from build123d import *

# Parameters (mm, degrees)
F0_R      = 25.4
F1_DEPTH  = 38.1
F3_R      = 4.1275
F4_DEPTH  = 20.0914
F5_R      = 3.4925
F6_DEPTH  = 18.0096
F7_W      = 5.08
F7_H      = 26.67
F8_DEPTH  = 5.08
F9_R      = 25.4
F9_R_2    = 4.1275
F10_DEPTH = 6.35
F11_R     = 25.4
F11_R_2   = 5.3975
F12_DEPTH = 12.7
F13_R     = 2.54
F14_DEPTH = 25.4
F16_R     = 22.225
F16_R_2   = 6.35
F17_DEPTH = 44.45


with BuildPart() as f1:
    # F0 (on Top) → F1 (new body)
    with BuildSketch(Plane.XY):
        Circle(F0_R)
    extrude(amount=-F1_DEPTH)

    # F3 (on face) → F4 (cut)
    with BuildSketch(Plane.XY):
        Circle(F3_R)
    extrude(amount=-F4_DEPTH, mode=Mode.SUBTRACT)

    # F5 (on face) → F6 (cut, through all)
    with BuildSketch(Plane.XY.offset(-20.0914)):
        Circle(F5_R)
    extrude(amount=-F6_DEPTH, mode=Mode.SUBTRACT)

    # F7 (on face) → F8 (cut)
    with BuildSketch(Plane(origin=(0, 0, -38.1), x_dir=(1, 0, 0), z_dir=(0, 0, -1))):
        with Locations((0, -13.335)):
            Rectangle(F7_W, F7_H)
    extrude(amount=-F8_DEPTH, mode=Mode.SUBTRACT)

    # F9 (on face) → F10 (join)
    with BuildSketch(Plane.XY):
        Circle(F9_R)
        Circle(F9_R_2, mode=Mode.SUBTRACT)
    extrude(amount=F10_DEPTH)

    # F11 (on face) → F12 (join)
    with BuildSketch(Plane.XY.offset(6.35)):
        Circle(F11_R)
        Circle(F11_R_2, mode=Mode.SUBTRACT)
    extrude(amount=F12_DEPTH)

    # F13 (on offset) → F14 (cut, through all)
    with BuildSketch(Plane.XZ.offset(-25.4)):
        with Locations((0, 1.524)):
            Circle(F13_R)
    extrude(amount=F14_DEPTH, mode=Mode.SUBTRACT)

    # F16 (on offset) → F17 (cut)
    with BuildSketch(Plane(origin=(0, 0, -31.75), x_dir=(1, 0, 0), z_dir=(0, 0, -1))):
        Circle(F16_R)
        Circle(F16_R_2, mode=Mode.SUBTRACT)
    extrude(amount=-F17_DEPTH, mode=Mode.SUBTRACT)


solid = f1.part
Read the model definition and answer for the solid it produces. Units are mm, in the model's axes. A direction names the side the tool comes from. Give positions to 0.01 mm unless a question says otherwise; leave off trailing zeros. Loops run counter-clockwise (first coordinate to the right, second up) from the corner with the lowest first, then second, coordinate; pieces in that order, holes last. Notation, with made-up numbers: (-36.75, 28.5) -> (21.25, 28.5) arc R8 ccw to (21.25, 38.5) -> close; hole circle Ø1 at (-18.75, 26). An arc over 180 degrees is marked (long way). Use a Markdown table: item, result.
Q1. A tool of negligible diameter and unlimited length cuts with its end or side. For faces 1 (the face through (2.346, 4.825, 0.551)), 2 (the face through (21.199, -6.676, -9.836)), 3 (the face through (2, -4, 6.35)), 4 (the face through (-0.8, -3.4, -29)), 5 (the face through (-2.54, 14, -36)), from which of +Z, -Z, +X, -X, +Y, -Y can it reach the whole face along a straight path? Write none if from no direction.
Solved:
| item | result |
|---|---|
| face 1 | +Y |
| face 2 | none |
| face 3 | +Z |
| face 4 | +Z, -Z |
| face 5 | -Z, +Y |
Q2. Determine the mould class of faces 6 (the face through (0, -5, -38.1)), 7 (the face through (0, 14, -33.02)), 8 (the face through (-5.506, -24.796, -9.925)) for opening direction X: pulls with the +X half, pulls with the -X half, needs draft (parallel to the pull), parting line crosses it, or undercut.
Solved:
| item | result |
|---|---|
| face 6 | needs draft |
| face 7 | undercut |
| face 8 | parting line crosses it |
Q3. Section D-D, the plane y = -10.5 is taken. Determine the outline of the cut face in (x, z).
Solved:
| item | result |
|---|---|
| outline | (-23.13, -38.1) -> (23.13, -38.1) -> (23.13, 19.05) -> (-23.13, 19.05) -> close; hole (-19.59, -31.75) -> (19.59, -31.75) -> (19.59, 12.7) -> (-19.59, 12.7) -> close |
Q4. Section A-A, the plane x = 0 is taken. Count the separate pieces of the cut face and the enclosed holes in it, then the cut area to 3 significant figures.
Solved:
| item | result |
|---|---|
| separate pieces | 3 |
| enclosed holes | 1 |
| area | 872 mm^2 |
Q5. Find the intervals of material crossed by line 1 along Z through (x, y) = (-20.5, -4); line 2 along Y through (x, z) = (1.5, -21); line 3 along Z through (x, y) = (0, 15), in increasing order.
Solved:
| item | result |
|---|---|
| line 1 | z = -38.1 to -31.75, 12.7 to 19.05 |
| line 2 | y = -25.36 to -22.17, -6.17 to -3.15, 3.15 to 6.17, 22.17 to 25.36 |
| line 3 | z = -33.02 to -31.75, 12.7 to 19.05 |
Q6. Each of these flat-tipped pins is pushed along its axis until it touches: pin 1 (4 mm diameter, centred on x = 1, y = -0.5, fed in from +Z); pin 2 (1.5 mm diameter, centred on x = 12, z = -11.5, fed in from -Y); pin 3 (4 mm diameter, centred on y = 13.5, z = -35, fed in from +X); pin 4 (3 mm diameter, centred on x = 2, y = 2, fed in from +Z). Where does it stop, or does it pass through?
Solved:
| item | result |
|---|---|
| pin 1 | passes through |
| pin 2 | stops at y = -22.77 |
| pin 3 | stops at x = 22.65 |
| pin 4 | stops at z = 6.35 |
